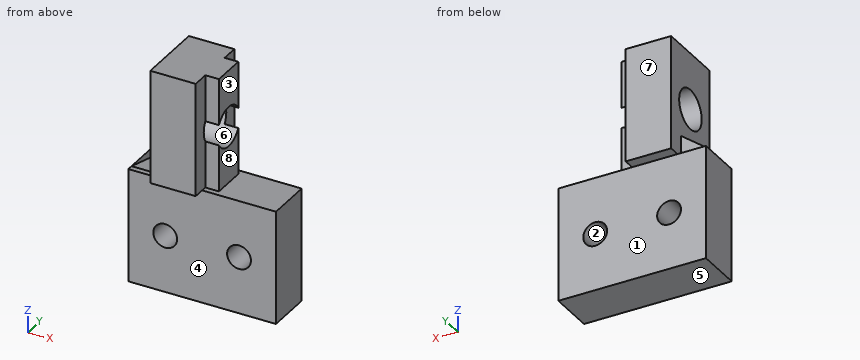
from build123d import *

# Parameters (mm, degrees)
SKETCH_2_W          = 13
SKETCH_2_H          = 10
SKETCH_2_R          = 1.05
EXTRUDE_1_DEPTH     = 6
EXTRUDE_2_DEPTH     = 10
SKETCH_4_W          = 13
SKETCH_4_H          = 10
CUT_EXTRUDE_1_DEPTH = 1
SKETCH_5_W          = 13
SKETCH_5_H          = 10
CUT_EXTRUDE_2_DEPTH = 1
SKETCH_6_R          = 1.75
CUT_EXTRUDE_3_DEPTH = 20.267848868
RIB_1_REACH         = 18.956
SKETCH_7_WALL_W     = 39.23500661
SKETCH_7_WALL_H     = 3


with BuildPart() as part:
    # 草图2 → 凸台-拉伸1 (new body)
    with BuildSketch(Plane(origin=(0, 0, 0), x_dir=(1, 0, 0), z_dir=(0, 1, 0))):
        Rectangle(SKETCH_2_W, SKETCH_2_H)
        with Locations(Location((-3.25, 0, 0), (0, 0, 270))):
            Circle(SKETCH_2_R, mode=Mode.SUBTRACT)
        with Locations(Location((3.25, 0, 0), (0, 0, 270))):
            Circle(SKETCH_2_R, mode=Mode.SUBTRACT)
    extrude(amount=EXTRUDE_1_DEPTH)

    # 草图3 → 凸台-拉伸2 (add)
    with BuildSketch(Plane.XY.offset(5)):
        Polygon((0, 6), (0, 4.5), (1.2, 4.5), (1.2, 1.5), (0, 1.5), (0, 0), (-4, 0), (-4, 6), align=None)
    extrude(amount=EXTRUDE_2_DEPTH)

    # 草图4 → 切除-拉伸1 (cut)
    with BuildSketch(Plane(origin=(0, 6, 0), x_dir=(1, 0, 0), z_dir=(0, 1, 0))):
        Rectangle(SKETCH_4_W, SKETCH_4_H)
    extrude(amount=-CUT_EXTRUDE_1_DEPTH, mode=Mode.SUBTRACT)

    # 草图5 → 切除-拉伸2 (cut)
    with BuildSketch(Plane.XZ):
        Rectangle(SKETCH_5_W, SKETCH_5_H)
    extrude(amount=-CUT_EXTRUDE_2_DEPTH, mode=Mode.SUBTRACT)

    # 草图6 → 切除-拉伸3 (cut, through all)
    with BuildSketch(Plane.ZY.offset(4)):
        with Locations((10, 3)):
            Circle(SKETCH_6_R)
    extrude(amount=-CUT_EXTRUDE_3_DEPTH, mode=Mode.SUBTRACT)

    # 草图7 wall → 筋1 (add, up to next)
    with BuildSketch(Plane(origin=(-5.172907339, 1.5, 6), x_dir=(0.798645937054, 0, 0.601801185798), z_dir=(-0.601801185798, 0, 0.798645937054)), mode=Mode.PRIVATE) as rib_1_sk1:
        with Locations((0, 1.5)):
            Rectangle(SKETCH_7_WALL_W, SKETCH_7_WALL_H)
    rib_1_tool1 = extrude(rib_1_sk1.sketch, amount=-RIB_1_REACH, mode=Mode.PRIVATE) - part.part
    add(rib_1_tool1.solids().sort_by_distance((-5.172907339, 1.5, 6))[0])


solid = part.part
Input: part model. Units: mm. Frame: model coordinates. Face numbers are marked on the shaded views. A direction names the side the tool comes from. Coordinates: 2 decimals unless noted, no trailing zeros. Write each loop counter-clockwise with the first axis right and the second up, starting at its lowest first coordinate (ties: lowest second). Pieces come first, ordered by that corner, then holes. Notation, with made-up numbers: M 31.5,72.5 L 43.5,72.5 A20 cw 43.5,101.5 Z; hole C 20,69 d7. An arc over 180 degrees is marked long. Answer as a JSON object with one key per item and string values. Group by question number.
(1) Section B-B on z = 0. Output: boundary loops of the cut face in (x, y).
(2) Set-up query: the marked faces 1, 2, 3, 4 and 5. Return all of +Z, -Z, +X, -X, +Y, -Y with unobstructed straight access to the full face (end or side cutting, diameter ignored); none if empty.
(3) Section C-C on y = 3. Output: boundary loops of the cut face in (x, z), plus the area to 3 significant figures.
(4) Section A-A on x = -3.25. Output: boundary loops of the cut face in (y, z).
(5) Mould query, pull axis Y, two halves, no side actions, for the marked faces 6, 7 and 8. Classes: pulls with the +Y half, pulls with the -Y half, needs draft (parallel to the pull), parting line crosses it, or undercut.
(6) Section D-D on z = 10. Output: boundary loops of the cut face in (x, y).
(7) Ray query, line 1 along Z through (x, y) = (-0.6, 3); line 2 along Z through (x, y) = (3.25, 1.9); line 3 along Z through (x, y) = (-3.25, 2.3). Return the intervals inside material, ascending. Write a range as [from, to].
(8) Contact query for flat-ended pins moving along their axis: P1, Ø2, axis at x = -5.5, z = 5.5, coming from the -Y side; P2, Ø1.5, axis at y = 1.5, z = 11, coming from the +X side; P3, Ø1.6, axis at y = 0.5, z = 11.5, coming from the +X side; P4, Ø1.5, axis at x = -1.5, z = 5, coming from the -Y side. Output: stop coordinate, or through.
Result set:
{
 "1": {"outline": "M -6.5,1 L -4.3,1 L -4.3,5 L -6.5,5 Z; M -2.2,1 L 2.2,1 L 2.2,5 L -2.2,5 Z; M 4.3,1 L 6.5,1 L 6.5,5 L 4.3,5 Z"},
 "2": {"face 1": "-Z, +X, -X, +Y", "face 2": "+Y, -Y", "face 3": "+Z, +X, +Y, -Y", "face 4": "-Z, +X, -X, -Y", "face 5": "-Z, +X, -X, +Y, -Y"},
 "3": {"outline": "M -6.5,-5 L 6.5,-5 L 6.5,5 L 1.2,5 L 1.2,8.25 L -4,8.25 L -4,6.88 L -6.5,5 Z; M -4,11.75 L 1.2,11.75 L 1.2,15 L -4,15 Z; hole C -3.25,0 d2.1; hole C 3.25,0 d2.1", "area": "159 mm2"},
 "4": {"outline": "M 0,5 L 1,5 L 1,1.05 L 5,1.05 L 5,5 L 6,5 L 6,15 L 0,15 Z; M 1,-5 L 5,-5 L 5,-1.05 L 1,-1.05 Z; hole C 3,10 d3.5"},
 "5": {"face 6": "undercut", "face 7": "pulls with the +Y half", "face 8": "needs draft"},
 "6": {"outline": "M -4,0 L 0,0 L 0,1.25 L -4,1.25 Z; M -4,4.75 L 0,4.75 L 0,6 L -4,6 Z"},
 "7": {"line 1": "z = [-5, 8.25], [11.75, 15]", "line 2": "z = [-5, -1.05], [1.05, 5]", "line 3": "z = [-5, -1.05], [1.05, 8.4], [11.6, 15]"},
 "8": {"P1": "stops at y = 1", "P2": "stops at x = 1.2", "P3": "stops at x = 0", "P4": "stops at y = 0"}
}
